```python
from build123d import *

# Parameters (mm, degrees)
F2_R     = 4.5
F3_DEPTH = 25


with BuildPart() as f1:
    # F0 (on Front) → F1 (revolve)
    with BuildSketch(Plane.XZ):
        Polygon((-8, 35), (0, 35), (8, 35), (8, 260), (35.5, 260), (35.5, 300), (0, 300), (-35.5, 300), (-35.5, 260), (-8, 260), align=None)
    revolve(axis=Axis((56.93949, 0, 0), (1, 0, 0)))

    # F2 (on face) → F3 (cut)
    with BuildSketch(Plane.YZ.offset(8)):
        with Locations((0, 65)):
            Circle(F2_R)
        with Locations((-65, 0)):
            Circle(F2_R)
        with Locations((0, -65)):
            Circle(F2_R)
        with Locations((65, 0)):
            Circle(F2_R)
    extrude(amount=-F3_DEPTH, mode=Mode.SUBTRACT)


solid = f1.part
```
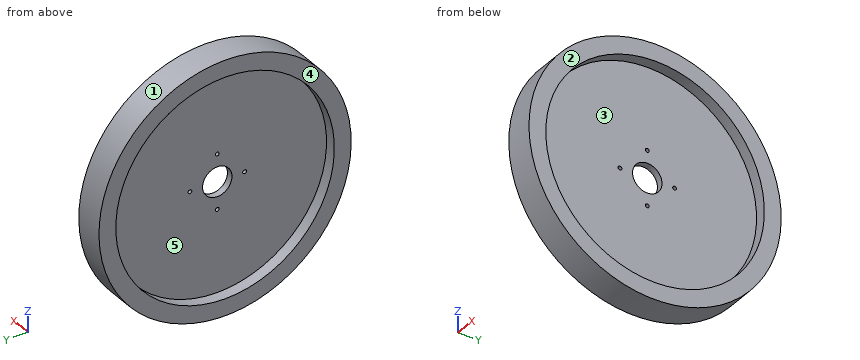
Check sheet for the modelled part. Datum: model origin and axes. Units: mm. Face numbers are marked on the shaded views. A direction names the side the tool comes from. Coordinates: 2 decimals unless noted, no trailing zeros. Loops run counter-clockwise (first coordinate to the right, second up) from the corner with the lowest first, then second, coordinate; pieces in that order, holes last.
1) Gauge pin test, flat ends, axial feed: pin 1 (8 mm diameter, centred on y = -65, z = 0, fed in from +X); pin 2 (3 mm diameter, centred on y = -142, z = 92.5, fed in from -X); pin 3 (8 mm diameter, centred on x = 23.5, y = -225.5, fed in from +Z); pin 4 (12 mm diameter, centred on y = 104, z = 181.5, fed in from +X). Record the tip position at first contact, or that the pin passes through.
2) Access from +Z, -Z, +X, -X, +Y, -Y to the whole of each face (thin tool, end or side, straight path). Record for the marked faces 4 and 5.
3) Sectioned sample at A-A (z = -250.5). Record the boundary of the cut face in (x, y).
4) Sectioned sample at B-B (y = 128). Record the boundary of the cut face in (x, z), and give its area (3 significant figures).
5) Release check for a two-part mould opening along Z. For the marked faces 1, 2 and 3 record: released by +Z, released by -Z, zero draft, split by the parting line, or undercut.
6) Material ranges on probe 1 along Z at (x, y) = (1.5, 0); probe 2 along X at (y, z) = (131, 214); probe 3 along Z at (x, y) = (-29, 0), recorded low to high.
Check sheet entries:
1. pin 1: passes through
1. pin 2: stops at x = -8
1. pin 3: stops at z = 202.33
1. pin 4: stops at x = 8
2. face 4: +Z, -Z, -X, +Y, -Y
2. face 5: -X
3. outline: (-35.5, -165.07) - (35.5, -165.07) - (35.5, -69.64) - (8, -69.64) - (8, 69.64) - (35.5, 69.64) - (35.5, 165.07) - (-35.5, 165.07) - (-35.5, 69.64) - (-8, 69.64) - (-8, -69.64) - (-35.5, -69.64) - close
4. outline: (-35.5, -271.32) - (35.5, -271.32) - (35.5, -226.31) - (8, -226.31) - (8, 226.31) - (35.5, 226.31) - (35.5, 271.32) - (-35.5, 271.32) - (-35.5, 226.31) - (-8, 226.31) - (-8, -226.31) - (-35.5, -226.31) - close
4. area: 13,600 mm2
5. face 1: split by the parting line
5. face 2: zero draft
5. face 3: undercut
6. probe 1: z = -300 to -69.5, -60.5 to -35, 35 to 60.5, 69.5 to 300
6. probe 2: x = -8 to 8
6. probe 3: z = -300 to -260, 260 to 300
